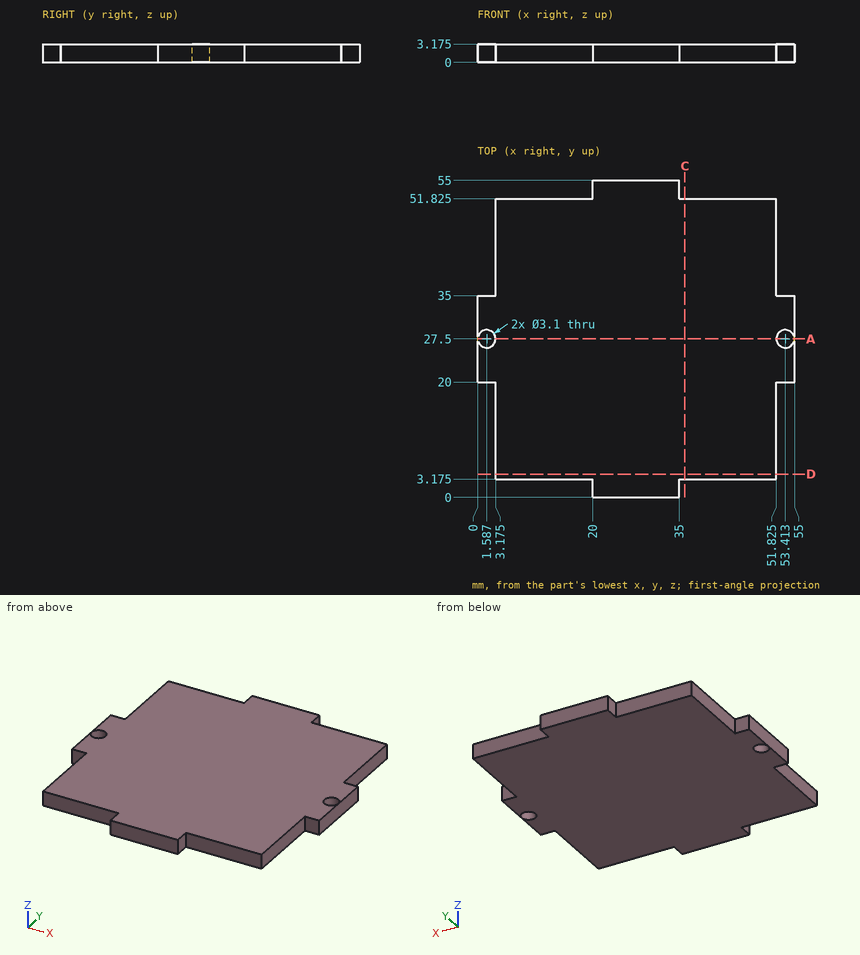
Geometry check sheet. Reference: drawing and pictorial views, mm from the part's lowest x, y, z. Give positions to 0.01 mm unless a question says otherwise; leave off trailing zeros. Write each loop counter-clockwise with the first axis right and the second up, starting at its lowest first coordinate (ties: lowest second). Pieces come first, ordered by that corner, then holes.
Item 1: Cross-section at A-A (y = 27.5). Count the separate pieces of the cut face and the enclosed holes in it, and give its area (3 significant figures).
Item 2: Gauge pin test, flat ends, axial feed: pin 1 (1.6 mm diameter, centred on y = 14.5, z = 1.5, fed in from -X) (1 decimal); pin 2 (1 mm diameter, centred on y = 53.5, z = 1.5, fed in from +X); pin 3 (1 mm diameter, centred on x = 53.5, z = 2.5, fed in from -Y). Record the tip position at first contact, or that the pin passes through.
Item 3: Scan lines: L1, parallel to X at y = 40.5, z = 0.7 (1 decimal); L2, parallel to X at y = 52, z = 2.55. Record each from-to range of solid material in increasing order.
Item 4: Cross-section at C-C (x = 36). Enter the section's corners in (y, z) (1 decimal).
Report:
1. separate pieces: 3
1. enclosed holes: 0
1. area: 155 mm2
2. pin 1: stops at x = 3.2
2. pin 2: stops at x = 35
2. pin 3: stops at y = 20
3. L1: x = 3.2 to 51.8
3. L2: x = 20 to 35
4. outline: (3.2, 0) - (51.8, 0) - (51.8, 3.2) - (3.2, 3.2) - close
